Geometry check sheet. Reference: the model listing, model coordinates, mm. Give positions to 0.01 mm unless a question says otherwise; leave off trailing zeros. Order: outer loops, then holes, each group sorted by start corner. A loop starts at its lowest first (then second) coordinate and runs counter-clockwise, first axis right, second up. Notation, with made-up numbers: M 69,57 L 99,57 A22 ccw 99,76 Z; hole C 69.5,-24.75 d3. An arc over 180 degrees is marked long. Use CSV: the item, a comma, the result in double quotes. Start each with the question number.
Autodesk Inventor part; units mm, degrees
ref_plane "YZ Plane" through (0, 0, 0) normal (1, 0, 0) x (0, 1, 0)
ref_plane "XZ Plane" through (0, 0, 0) normal (0, 1, 0) x (-1, 0, 0)
ref_plane "XY Plane" through (0, 0, 0) normal (0, 0, 1) x (1, 0, 0)
sketch "Sketch1" plane through (0, 0, 0) normal (1, 0, 0) x (0, 1, 0)
  line L0 (0, 0) -> (0, -250) construction
  circle A0 centre (0, -250) radius 5
  arc A1 (0, -17.5) -> (17.5, 0) centre (0, 0) ccw construction
  arc A2 (0, -232.5) -> (-17.5, -250) centre (0, -250) ccw construction
  line L1 (17.5, 0) -> (17.5, -250)
  line L2 (-17.5, 0) -> (-17.5, -250)
  arc A3 (-17.5, 0) -> (0, -17.5) centre (0, 0) ccw construction
  arc A4 (17.5, 0) -> (-17.5, 0) centre (0, 0) ccw
  arc A5 (17.5, -250) -> (0, -232.5) centre (0, -250) ccw construction
  arc A6 (-17.5, -250) -> (17.5, -250) centre (0, -250) ccw
  line L3 (0, 0) -> (0, -80) construction
  line L4 (0, -80) -> (5, -80) construction
  line L5 (5, -80) -> (5, -83)
  line L6 (5, -83) -> (-5, -83) construction
  line L7 (-5, -83) -> (-5, -80)
  line L8 (-5, -80) -> (0, -80) construction
  line L9 (0, -250) -> (0, -150) construction
  line L10 (0, -150) -> (5, -150) construction
  line L11 (5, -150) -> (5, -147)
  line L12 (5, -147) -> (-5, -147) construction
  line L13 (-5, -147) -> (-5, -150)
  line L14 (0, -150) -> (-5, -150) construction
  line L15 (7.5, 0) -> (7.5, -6) construction
  arc A7 (0, -7.25) -> (2.5, -6.8053) centre (0, 0) ccw construction
  line L16 (0, -7.25) -> (2.5, -7.25) construction
  line L17 (2.5, -7.25) -> (-2.5, -7.25) construction
  line L18 (-2.5, -7.25) -> (-2.5, -8.75)
  line L19 (-2.5, -8.75) -> (2.5, -8.75)
  line L20 (2.5, -8.75) -> (2.5, -7.25)
  line L21 (2.5, -7.25) -> (2.5, -6.8053)
  line L22 (-2.5, -7.25) -> (-2.5, -6.8053)
  arc A8 (-2.5, -6.8053) -> (0, -7.25) centre (0, 0) ccw construction
  arc A9 (2.5, -6.8053) -> (-2.5, -6.8053) centre (0, 0) ccw
  line L23 (0, -250) -> (7.75, -250) construction
  line L24 (7.75, -250) -> (7.75, -257.75) construction
  line L25 (7.75, -257.75) -> (0, -257.75) construction
  line L26 (0, -257.75) -> (0, -250) construction
  line L27 (7.75, -257.75) -> (-7.75, -257.75) construction
  line L28 (-7.75, -257.75) -> (-7.75, -242.25) construction
  line L29 (-7.75, -242.25) -> (7.75, -242.25) construction
  line L30 (7.75, -242.25) -> (7.75, -257.75) construction
  circle A10 centre (7.75, -242.25) radius 1.5
  circle A11 centre (7.75, -257.75) radius 1.5
  circle A12 centre (-7.75, -257.75) radius 1.5
  circle A13 centre (-7.75, -242.25) radius 1.5
  line L31 (5, -80) -> (5, -79.75)
  line L32 (5, -79.75) -> (-5, -79.75)
  line L33 (-5, -79.75) -> (-5, -80)
  line L34 (-5, -83) -> (-5, -83.25)
  line L35 (-5, -83.25) -> (5, -83.25)
  line L36 (5, -83.25) -> (5, -83)
  line L37 (-5, -147) -> (-5, -146.75)
  line L38 (-5, -146.75) -> (5, -146.75)
  line L39 (5, -146.75) -> (5, -147)
  line L40 (5, -150) -> (5, -150.25)
  line L41 (5, -150.25) -> (-5, -150.25)
  line L42 (-5, -150.25) -> (-5, -150)
  dimension "d1" = 250
  dimension "d2" = 10
  dimension "d3" = 35
  dimension "d4" = 35
  dimension "d5" = 80
  dimension "d6" = 5
  dimension "d7" = 3
  dimension "d9" = 100
  dimension "d10" = 3
  dimension "d14" = 10
  dimension "d27" = 2.5
  dimension "d28" = 5
  dimension "d29" = 1.5
  dimension "d30" = 7.25
  dimension "d31" = 7.75
  dimension "d32" = 7.75
  dimension "d33" = 15.5
  dimension "d34" = 15.5
  dimension "d35" = 3
  dimension "d36" = 3
  dimension "d37" = 3
  dimension "d38" = 3
  dimension "d39" = 64
  dimension "d40" = 0.25
  dimension "d41" = 10
  dimension "d42" = 0.25
  dimension "d43" = 0.25
  dimension "d44" = 10
  dimension "d45" = 0.25
  dimension "d46" = 0.25
  dimension "d47" = 10
  dimension "d48" = 0.25
  dimension "d49" = 0.25
  dimension "d50" = 10
  dimension "d51" = 0.25
extrude "Extrusion1" add sketch "Sketch1" along normal blind 3
properties part number "brazo1" material "PMMA Plastic"
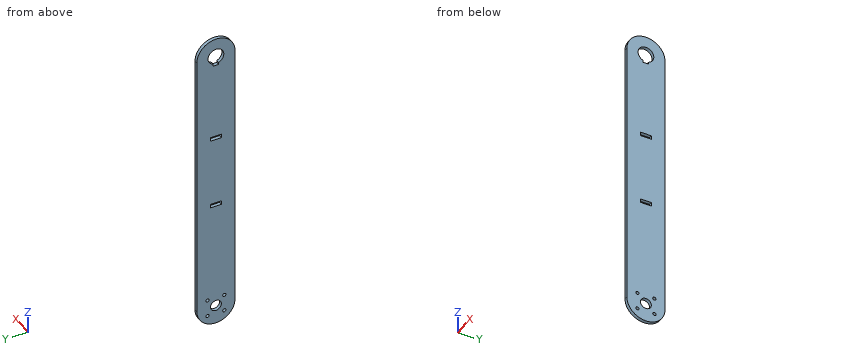
(1) Sectioned sample at D-D on y = 12. Record the cut outline in (x, z), then the cut area to 3 significant figures.
(2) Sectioned sample at B-B on x = 1.45. Give the number of separate pieces and of enclosed holes in the cut face, then the cut area to 3 significant figures.
(3) Thickness scan on line 1 (Z direction, x = 0.7, y = 0); line 2 (Y direction, x = 1.6, z = -242.25); line 3 (Z direction, x = 2, y = 7.75). Record the ranges inside material, lowest first.
(4) Sectioned sample at C-C on z = -2.5. Record the cut outline in (x, y).
(5) Sectioned sample at A-A on y = 0. Record the cut outline in (x, z).
(6) Go/stop test with flat-tipped pins: P1, Ø1.5, axis at x = 2, y = -2.5, coming from the -Z side; P2, Ø11.5, axis at y = 0, z = 0, coming from the +X side; P3, Ø3.5, axis at y = 7.75, z = -257.75, coming from the +X side. Record where each tip stops, or that it passes through.
Responses:
1,outline,"M 0,-262.74 L 3,-262.74 L 3,12.74 L 0,12.74 Z"
1,area,"826 mm2"
2,separate pieces,"1"
2,enclosed holes,"8"
2,area,"9,360 mm2"
3,line 1,"-267.5 to -255, -245 to -150.25, -146.75 to -83.25, -79.75 to -8.75, 7.25 to 17.5"
3,line 2,"-17.5 to -9.25, -6.25 to 6.25, 9.25 to 17.5"
3,line 3,"-265.69 to -259.25, -256.25 to -243.75, -240.75 to 15.69"
4,outline,"M 0,-17.5 L 3,-17.5 L 3,-6.81 L 0,-6.81 Z; M 0,6.81 L 3,6.81 L 3,17.5 L 0,17.5 Z"
5,outline,"M 0,-267.5 L 3,-267.5 L 3,-255 L 0,-255 Z; M 0,-245 L 3,-245 L 3,-150.25 L 0,-150.25 Z; M 0,-146.75 L 3,-146.75 L 3,-83.25 L 0,-83.25 Z; M 0,-79.75 L 3,-79.75 L 3,-8.75 L 0,-8.75 Z; M 0,7.25 L 3,7.25 L 3,17.5 L 0,17.5 Z"
6,P1,"z = -267.41"
6,P2,"through"
6,P3,"x = 3"
